Source: CAD feature listing. Evaluate the final solid. Frame: model axes, mm. Give positions to 0.01 mm unless a question says otherwise; leave off trailing zeros. Loops run counter-clockwise (first coordinate to the right, second up) from the corner with the lowest first, then second, coordinate; pieces in that order, holes last. Notation, with made-up numbers: (74, 37) -> (125, 37) arc R18 cw to (125, 71) -> close; hole circle Ø10 at (-10.75, 80). An arc over 180 degrees is marked (long way). Return JSON: item names as keys, results as strings. Group by question number.
```python
from build123d import *

# Parameters (mm, degrees)
ESQUISSE1_W             = 180
ESQUISSE1_H             = 430
BOSS_EXTRU_1_DEPTH      = 10
ESQUISSE2_W             = 146.172243306
ESQUISSE2_H             = 83.5
ENL_V_MAT_EXTRU_1_DEPTH = 10
ESQUISSE3_W             = 11.2
ESQUISSE3_H             = 46
ENL_V_MAT_EXTRU_2_DEPTH = 10


with BuildPart() as part:
    # Esquisse1 → Boss.-Extru.1 (new body)
    with BuildSketch(Plane(origin=(0, 0, 0), x_dir=(1, 0, 0), z_dir=(0, 1, 0))):
        with Locations((-90, 215)):
            Rectangle(ESQUISSE1_W, ESQUISSE1_H)
    extrude(amount=BOSS_EXTRU_1_DEPTH)

    # Esquisse2 → Enlèv. mat.-Extru.1 (cut)
    with BuildSketch(Plane(origin=(0, 10, 0), x_dir=(1, 0, 0), z_dir=(0, 1, 0))):
        with Locations((-88.713878322, 388.25)):
            Rectangle(ESQUISSE2_W, ESQUISSE2_H)
    extrude(amount=-ENL_V_MAT_EXTRU_1_DEPTH, mode=Mode.SUBTRACT)

    # Esquisse3 → Enlèv. mat.-Extru.2 (cut)
    with BuildSketch(Plane(origin=(0, 10, 0), x_dir=(1, 0, 0), z_dir=(0, 1, 0))):
        with Locations((-174.4, 407)):
            Rectangle(ESQUISSE3_W, ESQUISSE3_H)
        with Locations((-174.4, 23)):
            Rectangle(ESQUISSE3_W, ESQUISSE3_H)
    extrude(amount=-ENL_V_MAT_EXTRU_2_DEPTH, mode=Mode.SUBTRACT)


solid = part.part
```
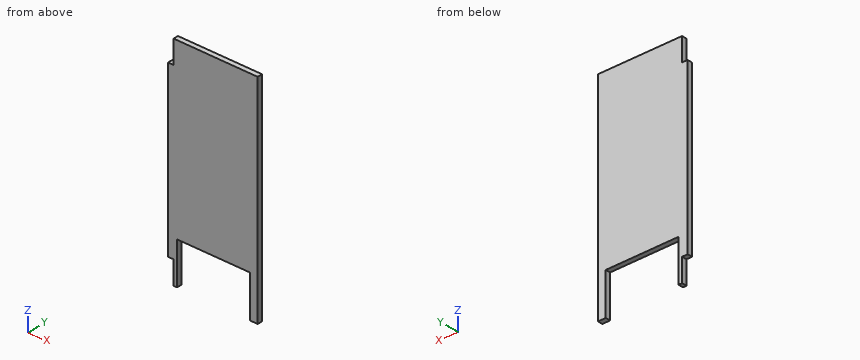
1) Contact query for flat-ended pins moving along their axis: P1, Ø3, axis at x = -174, y = 6.5, coming from the -Z side; P2, Ø3, axis at x = -32.5, y = 1.5, coming from the -Z side; P3, Ø5, axis at y = 5, z = -20, coming from the -X side. Output: stop coordinate, or through.
2) Cut plane C-C on x = -50.5. Return loops of the section in (y, z).
3) Material intervals for line 1 (X direction, y = 4.5, z = -391); line 2 (X direction, y = 4.75, z = -353); line 3 (Z direction, x = -42.5, y = 3), sorted ascending.
4) Cut plane A-A on z = -361. Return loops of the section in (x, y), then the cut area to 3 significant figures.
5) Cut plane B-B on y = 7. Return loops of the section in (x, z), then the cut area to 3 significant figures.
Calculated:
{
 "1": {"P1": "z = -384", "P2": "z = -346.5", "P3": "x = -168.8"},
 "2": {"outline": "(0, -346.5) -> (10, -346.5) -> (10, 0) -> (0, 0) -> close"},
 "3": {"line 1": "-168.8 to -161.8, -15.63 to 0", "line 2": "-180 to -161.8, -15.63 to 0", "line 3": "-346.5 to 0"},
 "4": {"outline": "(-180, 0) -> (-161.8, 0) -> (-161.8, 10) -> (-180, 10) -> close; (-15.63, 0) -> (0, 0) -> (0, 10) -> (-15.63, 10) -> close", "area": "338 mm2"},
 "5": {"outline": "(-180, -384) -> (-168.8, -384) -> (-168.8, -430) -> (-161.8, -430) -> (-161.8, -346.5) -> (-15.63, -346.5) -> (-15.63, -430) -> (0, -430) -> (0, 0) -> (-168.8, 0) -> (-168.8, -46) -> (-180, -46) -> close", "area": "64,200 mm2"}
}
